Check sheet for the modelled part. Datum: model origin and axes. Units: mm. A direction names the side the tool comes from. Round coordinates to 2 decimals unless told otherwise and drop trailing zeros. Loops run counter-clockwise (first coordinate to the right, second up) from the corner with the lowest first, then second, coordinate; pieces in that order, holes last. Notation, with made-up numbers: (-18, 13.25) - (36, 13.25) arc R28 ccw to (36, 50.25) - close; hole circle Ø6 at (45, 7.25). An arc over 180 degrees is marked (long way). Put each result on its own line as item: value. Start each with the question number.
Item 1: Section check A-A, the plane z = 7.5. Give the number of separate pieces and of enclosed holes in the cut face, and give its area (3 significant figures).
Item 2: Section check B-B, the plane y = -81. Record the cut outline in (x, z), and give its area (3 significant figures).
Item 3: Tool access check on faces 5 (the flat face through (79, -91, 0)), 6 (the flat face through (69.49, -77, 7)), 7 (the flat face through (70, -85.216, 7)), 8 (the flat face through (69.49, -94, -10)). Record the directions out of +Z, -Z, +X, -X, +Y, -Y that give a thin tool (end or side, any length) a straight path to the whole face; none if there is none.
Item 4: Gauge pin test, flat ends, axial feed: pin 1 Ø5.5 at (x, y) = (51.49, -84.32) entering from -Z; pin 2 Ø4.5 at (y, z) = (-81, 11) entering from +X; pin 3 Ø0.9 at (x, y) = (81, -91.5) entering from +Z; pin 4 Ø10 at (y, z) = (-77, -3.5) entering from -X. Record the tip position at first contact, or that the pin passes through.
Item 5: Section check C-C, the plane x = 63.5. Record the cut outline in (y, z), and give its area (3 significant figures).
Item 6: Draft check along X on faces 1 (the conical face through (42.565, -74.015, 14.886)), 2 (the cylindrical face through (49.886, -80, 2.761)), 3 (the cylindrical face through (68.588, -73.171, 7.402)), 4 (the cylindrical face through (51.051, -86.293, 7.198)). Enter one of: pulls with the +X half, pulls with the -X half, needs draft (parallel to the pull), parting line crosses it, or undercut.
Item 7: Material ranges on line 1 along Y through (x, z) = (75, -4); line 2 along Z through (x, y) = (67.5, -82); line 3 along Z through (x, y) = (48.5, -75.75), recorded low to high.
from build123d import *

# Parameters (mm, degrees)
SKETCH1_R           = 3.025
SKETCH1_R_2         = 2.025
BOSS_EXTRUDE1_DEPTH = 15
BOSS_EXTRUDE2_START = 5.6
SKETCH1_2_R         = 3.025
BOSS_EXTRUDE2_DEPTH = 9.4
BOSS_EXTRUDE3_DEPTH = 20
SKETCH2_R           = 2.65
CUT_EXTRUDE1_DEPTH  = 70
FILLET1_R           = 3
CHAMFER1_SIZE       = 0.4


# Some blends are built 0.0001 mm under size
with BuildPart() as part:
    # Sketch1 → Boss-Extrude1 (new body)
    with BuildSketch(Plane.XY):
        Polygon((66.489922843, -72.31585339), (69.489922843, -72.31585339), (69.489922843, -79.41585339), (70.989922843, -79.41585339), (70.989922843, -85.21585339), (69.489922843, -85.21585339), (69.489922843, -92.31585339), (76.589922843, -92.31585339), (82.389922843, -92.31585339), (89.489922843, -92.31585339), (89.489922843, -95.31585339), (66.489922843, -95.31585339), (41.489922843, -89.06585339), (41.489922843, -73.010297834), align=None)
        with Locations((48.489922843, -77.31585339)):
            Circle(SKETCH1_R, mode=Mode.SUBTRACT)
        with Locations((45.489922843, -84.31585339)):
            Circle(SKETCH1_R_2, mode=Mode.SUBTRACT)
        with Locations((51.489922843, -84.31585339)):
            Circle(SKETCH1_R_2, mode=Mode.SUBTRACT)
    extrude(amount=BOSS_EXTRUDE1_DEPTH)

    # Sketch1<2> → Boss-Extrude2 (add)
    with BuildSketch(Plane.XY.offset(BOSS_EXTRUDE2_START)):
        with Locations((48.489922843, -77.31585339)):
            Circle(SKETCH1_2_R)
    extrude(amount=BOSS_EXTRUDE2_DEPTH)

    # Sketch3 → Boss-Extrude3 (add)
    with BuildSketch(Plane(origin=(0, 0, 0), x_dir=(-1, 0, 0), z_dir=(0, 0, -1))):
        Polygon((-76.439922843, -92.31585339), (-69.489922843, -92.31585339), (-69.489922843, -95.31585339), (-89.489922843, -95.31585339), (-89.489922843, -92.31585339), (-82.539922843, -92.31585339), (-82.539922843, -89.31585339), (-76.439922843, -89.31585339), align=None)
    extrude(amount=BOSS_EXTRUDE3_DEPTH)

    # Sketch2 → Cut-Extrude1 (cut)
    with BuildSketch(Plane.XZ.offset(95.31585339)):
        with Locations(Location((79.489922843, 7.5, 0), (0, 0, 270))):
            Circle(SKETCH2_R)
    extrude(amount=-CUT_EXTRUDE1_DEPTH, mode=Mode.SUBTRACT)

    # Fillet1
    fillet1_edges = [part.edges().sort_by_distance(p)[0] for p in [
        (69.489922843, -72.31585339, 7.5),
        (41.489922843, -73.010297834, 7.5),
        (41.489922843, -89.06585339, 7.5),
    ]]
    fillet(fillet1_edges, radius=FILLET1_R - 0.0001)  # a hair under: the kernel refuses the full size

    # Chamfer1
    # the kernel refuses this chamfer: 0.4 mm, written as the material it takes off along each edge
    with BuildSketch(Plane(origin=(90.518596038, -95.31585339, 15), x_dir=(0, 0.9996219169112966, 0.02749587661058671), z_dir=(-1, 0, 0))) as chamfer1_piece_1:
        Polygon((CHAMFER1_SIZE * 0.999621916911, CHAMFER1_SIZE * 0.0274958766106), (-CHAMFER1_SIZE * 0.0274958766106, CHAMFER1_SIZE * 0.999621916911), (0, 0), align=None)
    extrude(amount=25.05734639, mode=Mode.SUBTRACT)
    with BuildSketch(Plane(origin=(89.489922843, -91.287180195, 15), x_dir=(-0.9996219169112966, 0, 0.02749587661058671), z_dir=(0, -1, 0))) as chamfer1_piece_2:
        Polygon((CHAMFER1_SIZE * 0.999621916911, CHAMFER1_SIZE * 0.0274958766106), (-CHAMFER1_SIZE * 0.0274958766106, CHAMFER1_SIZE * 0.999621916911), (0, 0), align=None)
    extrude(amount=5.05734639, mode=Mode.SUBTRACT)
    with BuildSketch(Plane(origin=(69.489922843, -92.31585339, 15), x_dir=(0, -0.9996219169112966, 0.02749587661058671), z_dir=(1, 0, 0))) as chamfer1_piece_3:
        Polygon((CHAMFER1_SIZE * 0.999621916911, CHAMFER1_SIZE * 0.0274958766106), (-CHAMFER1_SIZE * 0.0274958766106, CHAMFER1_SIZE * 0.999621916911), (0, 0), align=None)
    extrude(amount=21.028673195, mode=Mode.SUBTRACT)
    with BuildSketch(Plane(origin=(69.489922843, -85.21585339, 15), x_dir=(-0.9996219169112966, -2.1408261351483406e-13, 0.02749587661058671), z_dir=(0, -1, 0))) as chamfer1_piece_4:
        Polygon((CHAMFER1_SIZE * 0.999621916911, CHAMFER1_SIZE * 0.0274958766106), (-CHAMFER1_SIZE * 0.0274958766106, CHAMFER1_SIZE * 0.999621916911), (0, 0), align=None)
    extrude(amount=7.1, mode=Mode.SUBTRACT)
    with BuildSketch(Plane(origin=(45.489922843, -84.31585339, 15), x_dir=(1, 0, 0), z_dir=(0, -1, 0))) as chamfer1_piece_5:
        Polygon((2.025 + CHAMFER1_SIZE, 0), (2.025, -CHAMFER1_SIZE), (2.025, 0), align=None)
    revolve(axis=Axis((45.489922843, -84.31585339, 15), (0, 0, 1)), mode=Mode.SUBTRACT)
    with BuildSketch(Plane(origin=(72.018596038, -85.21585339, 15), x_dir=(0, 0.9996219169112966, 0.02749587661058671), z_dir=(-1, 0, 0)), Plane(origin=(69.489922843, -79.41585339, 15), x_dir=(0, -0.9996219169112966, 0.02749587661058671), z_dir=(1, 0, 0))) as chamfer1_piece_6:
        Polygon((CHAMFER1_SIZE * 0.999621916911, CHAMFER1_SIZE * 0.0274958766106), (-CHAMFER1_SIZE * 0.0274958766106, CHAMFER1_SIZE * 0.999621916911), (0, 0), align=None)
    extrude(amount=2.528673195, mode=Mode.SUBTRACT)
    with BuildSketch(Plane(origin=(51.489922843, -84.31585339, 15), x_dir=(1, 0, 0), z_dir=(0, -1, 0))) as chamfer1_piece_7:
        Polygon((2.025 + CHAMFER1_SIZE, 0), (2.025, -CHAMFER1_SIZE), (2.025, 0), align=None)
    revolve(axis=Axis((51.489922843, -84.31585339, 15), (0, 0, 1)), mode=Mode.SUBTRACT)
    with BuildSketch(Plane(origin=(70.989922843, -78.387180195, 15), x_dir=(-0.9996219169112966, -2.6206664757850423e-13, 0.02749587661058671), z_dir=(0, -1, 0))) as chamfer1_piece_8:
        Polygon((CHAMFER1_SIZE * 0.999621916911, CHAMFER1_SIZE * 0.0274958766106), (-CHAMFER1_SIZE * 0.0274958766106, CHAMFER1_SIZE * 0.999621916911), (0, 0), align=None)
    extrude(amount=7.85734639, mode=Mode.SUBTRACT)
    with BuildSketch(Plane(origin=(44.406524418, -72.929281124, 15), x_dir=(-0.0007634798546782339, 0.027485274768416574, -0.9996219169112971), z_dir=(0.9996144206527183, 0.027767067240353136, 0))) as chamfer1_piece_9:
        Polygon((CHAMFER1_SIZE * 0.999621916911, -CHAMFER1_SIZE * 0.0274958766106), (-CHAMFER1_SIZE * 0.0274958766106, -CHAMFER1_SIZE * 0.999621916911), (0, 0), align=None)
    extrude(amount=23.120589807, mode=Mode.SUBTRACT)
    with BuildSketch(Plane(origin=(69.489922843, -75.31575339, 15), x_dir=(-0.9996219169112966, 2.140826135148345e-13, 0.02749587661058671), z_dir=(0, -1, 0))) as chamfer1_piece_10:
        Polygon((CHAMFER1_SIZE * 0.999621916911, CHAMFER1_SIZE * 0.0274958766106), (-CHAMFER1_SIZE * 0.0274958766106, CHAMFER1_SIZE * 0.999621916911), (0, 0), align=None)
    extrude(amount=4.1001, mode=Mode.SUBTRACT)
    with BuildSketch(Plane(origin=(41.489922843, -86.723602248, 15), x_dir=(0.9996219169112966, 0, 0.027495876610587656), z_dir=(0, 1, 0))) as chamfer1_piece_11:
        Polygon((CHAMFER1_SIZE * 0.999621916911, CHAMFER1_SIZE * 0.0274958766106), (-CHAMFER1_SIZE * 0.0274958766106, CHAMFER1_SIZE * 0.999621916911), (0, 0), align=None)
    extrude(amount=10.795577824, mode=Mode.SUBTRACT)
    with BuildSketch(Plane(origin=(67.487882428, -95.565343286, 15), x_dir=(0.24244392641809726, 0.9697757056723949, 0.027495876610587038), z_dir=(-0.9701425001453322, 0.2425356250363316, 0))) as chamfer1_piece_12:
        Polygon((CHAMFER1_SIZE * 0.999621916911, CHAMFER1_SIZE * 0.0274958766106), (-CHAMFER1_SIZE * 0.0274958766106, CHAMFER1_SIZE * 0.999621916911), (0, 0), align=None)
    extrude(amount=24.455832214, mode=Mode.SUBTRACT)
    with BuildSketch(Plane(origin=(44.489822843, -86.723602248, 15), x_dir=(-1, 0, 0), z_dir=(0, 1, 0))) as chamfer1_piece_13:
        Polygon((2.9999 - CHAMFER1_SIZE, 0), (2.9999, -CHAMFER1_SIZE), (2.9999, 0), align=None)
    revolve(axis=Axis((44.489822843, -86.723602248, 15), (0, 0, 1)), revolution_arc=75.963756532, mode=Mode.SUBTRACT)
    with BuildSketch(Plane(origin=(44.489822843, -75.928024424, 15), x_dir=(-0.02776706724035276, 0.9996144206527183, 0), z_dir=(0.9996144206527183, 0.02776706724035276, 0))) as chamfer1_piece_14:
        Polygon((2.9999 - CHAMFER1_SIZE, 0), (2.9999, -CHAMFER1_SIZE), (2.9999, 0), align=None)
    revolve(axis=Axis((44.489822843, -75.928024424, 15), (0, 0, 1)), revolution_arc=88.408859729, mode=Mode.SUBTRACT)
    with BuildSketch(Plane(origin=(66.490022843, -75.31575339, 15), x_dir=(0, 1, 0), z_dir=(-1, 0, 0))) as chamfer1_piece_15:
        Polygon((2.9999, CHAMFER1_SIZE), (2.9999 - CHAMFER1_SIZE, 0), (2.9999, 0), align=None)
    revolve(axis=Axis((66.490022843, -75.31575339, 15), (0, 0, -1)), revolution_arc=90, mode=Mode.SUBTRACT)
    with BuildSketch(Plane(origin=(65.461249648, -72.31585339, 15), x_dir=(0, 0.027495876610595927, -0.9996219169112964), z_dir=(1, 0, 0))) as chamfer1_piece_16:
        Polygon((CHAMFER1_SIZE * 0.999621916911, -CHAMFER1_SIZE * 0.0274958766106), (-CHAMFER1_SIZE * 0.0274958766106, -CHAMFER1_SIZE * 0.999621916911), (0, 0), align=None)
    extrude(amount=1.028773195, mode=Mode.SUBTRACT)
    with BuildSketch(Plane(origin=(69.489922843, -85.21585339, 15), x_dir=(-0.9996219169112966, -2.1408261351483406e-13, 0.02749587661058671), z_dir=(0, -1, 0))) as chamfer1_piece_17a_section:
        Polygon((CHAMFER1_SIZE * 0.999621916911, CHAMFER1_SIZE * 0.0274958766106), (-CHAMFER1_SIZE * 0.0274958766106, CHAMFER1_SIZE * 0.999621916911), (0, 0), align=None)
    chamfer1_piece_17a = extrude(amount=8.128673195, mode=Mode.PRIVATE)
    chamfer1_piece_17a = split(chamfer1_piece_17a, bisect_by=Plane(origin=(69.358005392, -92.31585339, 14.868082549), z_dir=(0, -1, 0)), keep=Keep.TOP, mode=Mode.PRIVATE)
    with BuildSketch(Plane(origin=(68.461249648, -92.31585339, 15), x_dir=(0, -0.9996219169112966, 0.02749587661058671), z_dir=(1, 0, 0))) as chamfer1_piece_17b_section:
        Polygon((CHAMFER1_SIZE * 0.999621916911, CHAMFER1_SIZE * 0.0274958766106), (-CHAMFER1_SIZE * 0.0274958766106, CHAMFER1_SIZE * 0.999621916911), (0, 0), align=None)
    chamfer1_piece_17b = extrude(amount=22.05734639, mode=Mode.PRIVATE)
    chamfer1_piece_17b = split(chamfer1_piece_17b, bisect_by=Plane(origin=(69.489922843, -92.44777084, 14.868082549), z_dir=(-1, 0, 0)), keep=Keep.TOP, mode=Mode.PRIVATE)
    chamfer1_piece_17 = chamfer1_piece_17a & chamfer1_piece_17b
    add(chamfer1_piece_17, mode=Mode.SUBTRACT)
    with BuildSketch(Plane(origin=(72.018596038, -85.21585339, 15), x_dir=(0, 0.9996219169112966, 0.02749587661058671), z_dir=(-1, 0, 0))) as chamfer1_piece_18a_section:
        Polygon((CHAMFER1_SIZE * 0.999621916911, CHAMFER1_SIZE * 0.0274958766106), (-CHAMFER1_SIZE * 0.0274958766106, CHAMFER1_SIZE * 0.999621916911), (0, 0), align=None)
    chamfer1_piece_18a = extrude(amount=3.55734639, mode=Mode.PRIVATE)
    chamfer1_piece_18a = split(chamfer1_piece_18a, bisect_by=Plane(origin=(69.489922843, -85.083935939, 14.868082549), z_dir=(-1, 0, 0)), keep=Keep.TOP, mode=Mode.PRIVATE)
    with BuildSketch(Plane(origin=(69.489922843, -84.187180195, 15), x_dir=(-0.9996219169112966, -2.1408261351483406e-13, 0.02749587661058671), z_dir=(0, -1, 0))) as chamfer1_piece_18b_section:
        Polygon((CHAMFER1_SIZE * 0.999621916911, CHAMFER1_SIZE * 0.0274958766106), (-CHAMFER1_SIZE * 0.0274958766106, CHAMFER1_SIZE * 0.999621916911), (0, 0), align=None)
    chamfer1_piece_18b = extrude(amount=8.128673195, mode=Mode.PRIVATE)
    chamfer1_piece_18b = split(chamfer1_piece_18b, bisect_by=Plane(origin=(69.358005392, -85.21585339, 14.868082549), z_dir=(0, 1, 0)), keep=Keep.TOP, mode=Mode.PRIVATE)
    chamfer1_piece_18 = chamfer1_piece_18a & chamfer1_piece_18b
    add(chamfer1_piece_18, mode=Mode.SUBTRACT)
    with BuildSketch(Plane(origin=(69.489922843, -75.31575339, 15), x_dir=(-0.9996219169112966, 2.140826135148345e-13, 0.02749587661058671), z_dir=(0, -1, 0))) as chamfer1_piece_19a_section:
        Polygon((CHAMFER1_SIZE * 0.999621916911, CHAMFER1_SIZE * 0.0274958766106), (-CHAMFER1_SIZE * 0.0274958766106, CHAMFER1_SIZE * 0.999621916911), (0, 0), align=None)
    chamfer1_piece_19a = extrude(amount=5.128773195, mode=Mode.PRIVATE)
    chamfer1_piece_19a = split(chamfer1_piece_19a, bisect_by=Plane(origin=(69.358005392, -79.41585339, 14.868082549), z_dir=(0, -1, 0)), keep=Keep.TOP, mode=Mode.PRIVATE)
    with BuildSketch(Plane(origin=(68.461249648, -79.41585339, 15), x_dir=(0, -0.9996219169112966, 0.02749587661058671), z_dir=(1, 0, 0))) as chamfer1_piece_19b_section:
        Polygon((CHAMFER1_SIZE * 0.999621916911, CHAMFER1_SIZE * 0.0274958766106), (-CHAMFER1_SIZE * 0.0274958766106, CHAMFER1_SIZE * 0.999621916911), (0, 0), align=None)
    chamfer1_piece_19b = extrude(amount=3.55734639, mode=Mode.PRIVATE)
    chamfer1_piece_19b = split(chamfer1_piece_19b, bisect_by=Plane(origin=(69.489922843, -79.54777084, 14.868082549), z_dir=(-1, 0, 0)), keep=Keep.TOP, mode=Mode.PRIVATE)
    chamfer1_piece_19 = chamfer1_piece_19a & chamfer1_piece_19b
    add(chamfer1_piece_19, mode=Mode.SUBTRACT)


solid = part.part
Check result:
1. separate pieces: 2
1. enclosed holes: 2
1. area: 579 mm²
2. outline: (41.49, 0) - (70.99, 0) - (70.99, 14.6) - (70.59, 15) - (41.89, 15) - (41.49, 14.6) - close
2. area: 442 mm²
3. face 5: +Z, +X, +Y
3. face 6: +Z, -Z, +X, +Y
3. face 7: +Z, -Z, +X
3. face 8: -Z, -X, +Y, -Y
4. pin 1: z = 0
4. pin 2: x = 70.99
4. pin 3: z = 0
4. pin 4: x = 41.49
5. outline: (-94.57, 0) - (-72.4, 0) - (-72.4, 14.6) - (-72.8, 15) - (-94.16, 15) - (-94.57, 14.6) - close
5. area: 332 mm²
6. face 1: pulls with the -X half
6. face 2: undercut
6. face 3: pulls with the +X half
6. face 4: undercut
7. line 1: -95.32 to -92.32
7. line 2: 0 to 15
7. line 3: 5.6 to 15
